CAD build for the part. Positions are in the model's coordinates, mm. A direction names the side the tool comes from. Coordinates: 2 decimals unless noted, no trailing zeros. Loops run counter-clockwise (first coordinate to the right, second up) from the corner with the lowest first, then second, coordinate; pieces in that order, holes last.
1) Two-plate mould, pull along Z, no slides. Class faces 1 (the flat face through (-4.762, 0, 0)), 2 (the flat face through (0.762, -7, 0)), 3 (the cylindrical face through (0.376, 27.933, -0.614)): +Z half, -Z half, draft (parallel to the pull), parting line (faces both ways), or undercut.
2) Saw through at D-D, the plane y = 19.5. Write the cut outline in (x, z), and give its area (3 significant figures).
3) Wall check: line 1 along Z through (x, y) = (-3.15, 0); line 2 along X through (y, z) = (19, 7); line 3 along Y through (x, z) = (-4, -1). Give the ranges that are in metal, low to high.
4) Which spindle directions (+Z, -Z, +X, -X, +Y, -Y) get a long thin tool onto all of the face, cutting with end or side? Do faces 4 (the cylindrical face through (-1.96, -0.28, 2.11)), 5 (the cylindrical face through (-3.131, 0.633, -2.852)), 6 (the flat face through (-6.35, 0, 0)). Say none if no direction does.
5) Saw through at B-B, the plane x = -3.75. Write the cut outline in (y, z).
6) Saw through at A-A, the plane z = 0. Write the cut outline in (x, y), and give its area (3 significant figures).
7) Saw through at C-C, the plane y = -12. Write the cut outline in (x, z), and give its area (3 significant figures).
8) Pin check, flat tips, straight feed: pin 1 Ø17 at (y, z) = (10.5, -5) entering from -X; pin 2 Ø1.5 at (x, z) = (-1.5, -7) entering from -Y. Stop position of each tip, or through.
```python
from build123d import *

# Parameters (mm, degrees)
F1_DEPTH = 0.762
F2_R     = 2.921
F3_DEPTH = 6.35
F4_R     = 2.12725
F5_DEPTH = 5.5245


with BuildPart() as f1:
    # F0 (on Right) → F1 (new body)
    with BuildSketch(Plane.YZ):
        with BuildLine():
            Line((-27.94, -27.94), (0, -27.94))
            ThreePointArc((0, -27.94), (27.94, 0), (0, 27.94))
            Line((0, 27.94), (-27.94, 27.94))
            Line((-27.94, 27.94), (-27.94, -27.94))
        make_face()
    extrude(amount=F1_DEPTH)

    # F2 (on face) → F3 (join)
    with BuildSketch(Plane(origin=(0, 0, 0), x_dir=(0, -1, 0), z_dir=(-1, 0, 0))):
        Circle(F2_R)
    extrude(amount=F3_DEPTH)

    # F4 (on face) → F5 (cut)
    with BuildSketch(Plane.YZ.offset(0.762)):
        Circle(F4_R)
    extrude(amount=-F5_DEPTH, mode=Mode.SUBTRACT)


solid = f1.part
```
Data:
1. face 1: undercut
1. face 2: draft
1. face 3: parting line
2. outline: (0, -20.01) - (0.76, -20.01) - (0.76, 20.01) - (0, 20.01) - close
2. area: 30.5 mm2
3. line 1: z = -2.92 to -2.13, 2.13 to 2.92
3. line 2: x = 0 to 0.76
3. line 3: y = -2.74 to -1.88, 1.88 to 2.74
4. face 4: +X
4. face 5: -X
4. face 6: +Z, -Z, -X, +Y, -Y
5. outline: circle Ø5.84 at (0, 0); hole circle Ø4.25 at (0, 0)
6. outline: (-6.35, -2.92) - (0, -2.92) - (0, -27.94) - (0.76, -27.94) - (0.76, -2.13) - (-4.76, -2.13) - (-4.76, 2.13) - (0.76, 2.13) - (0.76, 27.94) - (0, 27.94) - (0, 2.92) - (-6.35, 2.92) - close
6. area: 56.2 mm2
7. outline: (0, -27.94) - (0.76, -27.94) - (0.76, 27.94) - (0, 27.94) - close
7. area: 42.6 mm2
8. pin 1: stops at x = 0
8. pin 2: passes through
